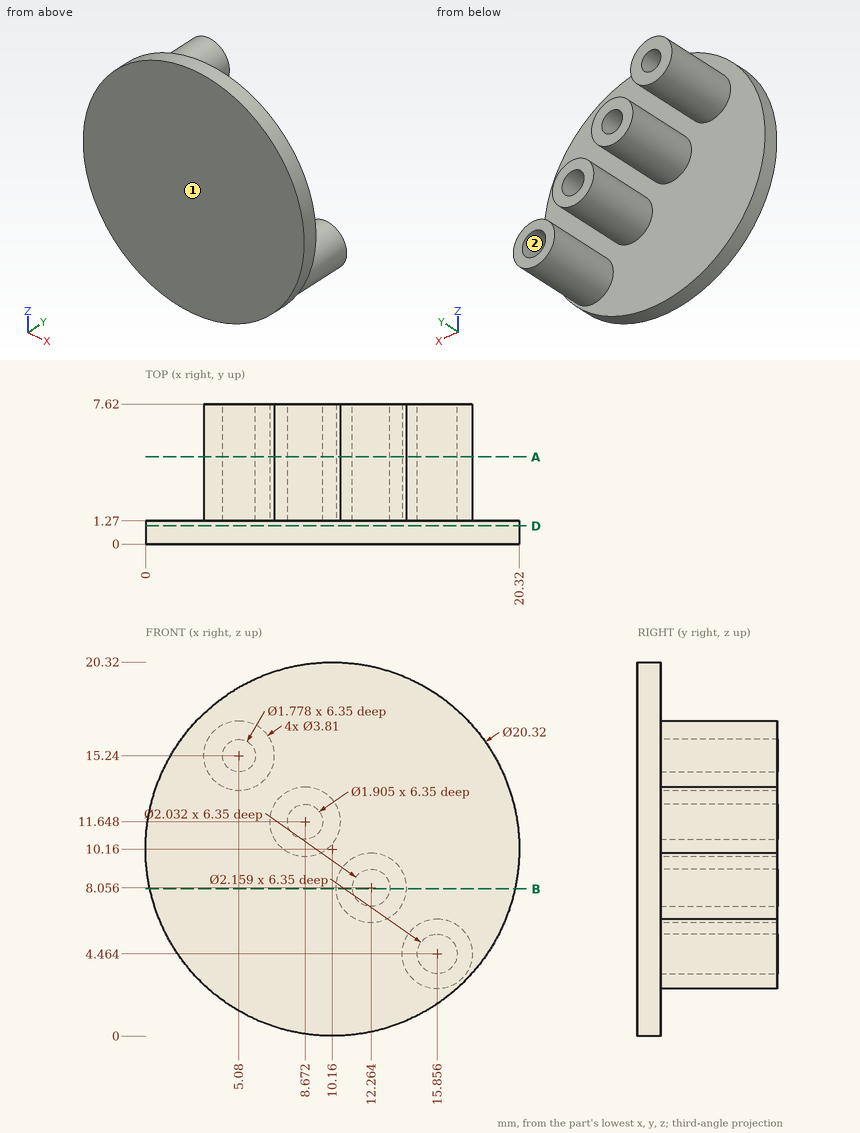
Verification items for this drawing (mm, ordinates from the low corner). Coordinates: 2 decimals unless noted, no trailing zeros. Order: outer loops, then holes, each group sorted by start corner. A loop starts at its lowest first (then second) coordinate and runs counter-clockwise, first axis right, second up. Notation, with made-up numbers: M 77,40 L 101,40 A31 ccw 101,70 Z; hole C 59.25,64 d9. An arc over 180 degrees is marked long. Answer as a JSON object with one key per item and string values.
Q1. Cross-section at B-B on z = 8. Record the cut outline in (x, y).
Results are:
{"outline": "M 0.23,0 L 20.09,0 L 20.09,1.27 L 14.17,1.27 L 14.17,7.62 L 13.28,7.62 L 13.28,1.27 L 11.25,1.27 L 11.25,7.62 L 10.36,7.62 L 10.36,1.27 L 0.23,1.27 Z"}
Q2. Cross-section at A-A on y = 4.75. Record the cut outline in (x, z) (1 decimal).
Results are:
{"outline": "C 5.1,15.2 d3.8; C 8.7,11.6 d3.8; C 12.3,8.1 d3.8; C 15.9,4.5 d3.8; hole C 5.1,15.2 d1.8; hole C 8.7,11.6 d1.9; hole C 12.3,8.1 d2; hole C 15.9,4.5 d2.2"}
Q3. Release check for a two-part mould opening along X. For the marked faces 1 and 2 record: released by +X, released by -X, zero draft, split by the parting line, or undercut.
Results are:
{"face 1": "zero draft", "face 2": "undercut"}
Q4. Cross-section at D-D on y = 1. Record the cut outline in (x, z).
Results are:
{"outline": "C 10.16,10.16 d20.32"}
Q5. Depth check by flat-ended pin: pin 1 Ø0.5 at (x, z) = (5, 15.5) entering from +Y; pin 2 Ø2 at (y, z) = (1.5, 17.5) entering from -X; pin 3 Ø3 at (y, z) = (5, 8.5) entering from -X (1 decimal). Enter the tip coordinate at first touch or a pass-through.
Results are:
{"pin 1": "stops at y = 1.27", "pin 2": "stops at x = 2.24", "pin 3": "stops at x = 7.7"}
Q6. Scan lines: line 1 (X direction, y = 4.75, z = 15.24) (1 decimal); line 2 (Y direction, x = 1, z = 12.5); line 3 (X direction, y = 5, z = 8.25). Record each from-to range of solid material in increasing order.
Results are:
{"line 1": "x = 3.2 to 4.2, 6 to 7", "line 2": "y = 0 to 1.27", "line 3": "x = 10.37 to 11.27, 13.26 to 14.16"}
